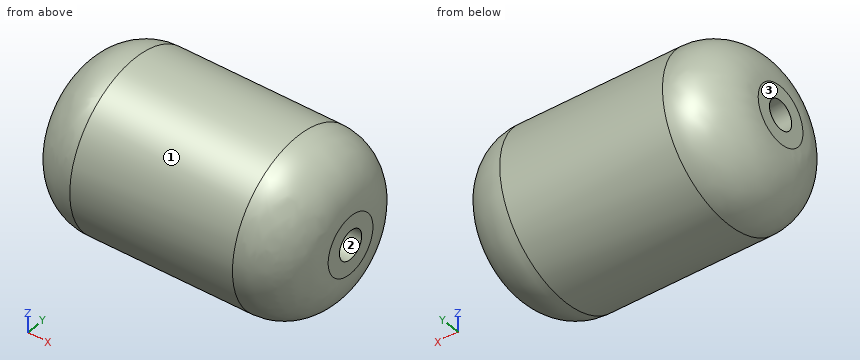
from build123d import *


with BuildPart() as part:
    # Sketch1 → Revolve1 (revolve)
    with BuildSketch(Plane.XY):
        with BuildLine():
            Line((-100, 21.579100204), (-100, 10.707094489))
            Line((-100, 10.707094489), (100, 10.707094489))
            Line((100, 10.707094489), (100, 21.579100204))
            ThreePointArc((100, 21.579100204), (88.284271247, 49.863371451), (60, 61.579100204))
            Line((60, 61.579100204), (-60, 61.579100204))
            ThreePointArc((-60, 61.579100204), (-88.284271247, 49.863371451), (-100, 21.579100204))
        make_face()
        with BuildLine():
            Line((-97.46, 21.579100204), (-97.46, 13.247094489))
            Line((-97.46, 13.247094489), (97.46, 13.247094489))
            Line((97.46, 13.247094489), (97.46, 21.579100204))
            ThreePointArc((97.46, 21.579100204), (86.488220023, 48.067320227), (60, 59.039100204))
            Line((60, 59.039100204), (-60, 59.039100204))
            ThreePointArc((-60, 59.039100204), (-86.488220023, 48.067320227), (-97.46, 21.579100204))
        make_face(mode=Mode.SUBTRACT)
    revolve(axis=Axis((0, 0, 0), (-1, 0, 0)))


solid = part.part
The listing builds one solid part. Answer for the finished solid, in the listing's coordinates (mm). Face numbers are marked on the shaded views. Coordinates: 2 decimals unless noted, no trailing zeros. Write each loop counter-clockwise with the first axis right and the second up, starting at its lowest first coordinate (ties: lowest second). Pieces come first, ordered by that corner, then holes. Notation, with made-up numbers: (56.25, -5) - (60.25, -5) arc R14 cw to (60.25, 8) - close; hole circle Ø2 at (57, 12). An arc over 180 degrees is marked (long way). Return JSON: item names as keys, results as strings.
1. Consider line 1 along Y through (x, z) = (16, 0); line 2 along Z through (x, y) = (-66.5, 2.5). Determine where each line is inside the solid, lowest interval first.
Final values:
{"line 1": "-61.58 to -59.04, -13.25 to -10.71, 10.71 to 13.25, 59.04 to 61.58", "line 2": "-61 to -58.42, -13.01 to -10.41, 10.41 to 13.01, 58.42 to 61"}
2. Each of these flat-tipped pins is pushed along its axis until it touches: pin 1 Ø6 at (y, z) = (-22.5, -16.5) entering from -X; pin 2 Ø5 at (x, y) = (-59, -4.5) entering from +Z; pin 3 Ø12 at (x, y) = (3, 42.5) entering from +Z; pin 4 Ø12 at (x, z) = (-36.5, 6) entering from -Y. Where does it stop, or does it pass through?
Final values:
{"pin 1": "x = -99.86", "pin 2": "z = 61.55", "pin 3": "z = 49.6", "pin 4": "y = -61.58"}
3. For a pull along Z with two mould halves and no side action, classify the marked faces 1, 2 and 3 as +Z half, -Z half, draft (parallel to the pull), parting line (faces both ways), or undercut.
Final values:
{"face 1": "parting line", "face 2": "undercut", "face 3": "draft"}
4. The part is cut by section A-A on z = 0. Count the separate pieces of the cut face and the enclosed holes in it, then the cut area to 3 significant figures.
Final values:
{"separate pieces": "2", "enclosed holes": "2", "area": "2,330 mm^2"}
5. The part is cut by section C-C on x = 1.5. Determine the outline of the cut face in (y, z), then the cut area to 3 significant figures.
Final values:
{"outline": "circle Ø123.16 at (0, 0); circle Ø26.49 at (0, 0); hole circle Ø118.08 at (0, 0); hole circle Ø21.41 at (0, 0)", "area": "1,150 mm^2"}
